Part model, mm, in its own coordinate system. A direction names the side the tool comes from. Coordinates: 2 decimals unless noted, no trailing zeros. Order: outer loops, then holes, each group sorted by start corner. A loop starts at its lowest first (then second) coordinate and runs counter-clockwise, first axis right, second up.
1) Cut at A-A (x = 0). List the corners of the cut face in (y, z).
2) Mould opens along Z. For faces 4 (the flat face through (4, -1, -9)), 5 (the cylindrical face through (-1.73, 2.03, 7.81)), 6 (the cylindrical face through (11.923, 1.535, 3.755)) say: +Z half, -Z half, draft (parallel to the pull), parting line (faces both ways), or undercut.
3) Cut at D-D (z = -3.25). List the corners of the cut face in (x, y), and give its area (3 significant figures).
4) Pin check, flat tips, straight feed: pin 1 Ø1.6 at (x, z) = (-9, -6.5) entering from +Y; pin 2 Ø9.5 at (x, z) = (0, 0) entering from -Y; pin 3 Ø3 at (x, y) = (4.5, 3) entering from -Z; pin 4 Ø2 at (y, z) = (3, 3.5) entering from +X. Stop position of each tip, or through.
5) Tool access for faces 1 (the flat face through (11, 0, 0)), 2 (the flat face through (-0.2, 4, 8.2)), 3 (the flat face through (-2, 0, -8)): list every direction of +Z, -Z, +X, -X, +Y, -Y with a clear straight run to the whole face (end or side of a thin tool).
6) Cut at B-B (z = 0). List the corners of the cut face in (x, y), and give its area (3 significant figures).
7) Wall check: L1, parallel to X at y = 1.95, z = 0; L2, parallel to Z at x = 0, y = 2.25; L3, parallel to X at y = 0.8, z = -0.75. Give the ranges that are in metal, low to high.
8) Cut at C-C (y = 0.35). List the corners of the cut face in (x, z).
```python
from build123d import *

# Parameters (mm, degrees)
SKETCH_1_R          = 12.5
EXTRUDE_1_DEPTH     = 4
SKETCH_2_R          = 1
EXTRUDE_2_DEPTH     = 7.5
SKETCH_5_R          = 6
CUT_EXTRUDE_1_DEPTH = 10
SKETCH_7_R          = 1
CUT_EXTRUDE_2_DEPTH = 7.5
SKETCH_8_R          = 12.5
SKETCH_8_R_2        = 6
CUT_EXTRUDE_3_DEPTH = 10
SKETCH_9_R          = 1
EXTRUDE_3_DEPTH     = 10
SKETCH_10_R         = 1
CUT_EXTRUDE_4_DEPTH = 14
SKETCH_11_R         = 8
CUT_EXTRUDE_5_DEPTH = 10
SKETCH_13_R         = 12.5
SKETCH_13_R_2       = 9.6
EXTRUDE_5_DEPTH     = 1


with BuildPart() as part:
    # 草图1 → 凸台-拉伸1 (new body)
    with BuildSketch(Plane(origin=(0, 0, 0), x_dir=(1, 0, 0), z_dir=(0, 1, 0))):
        Circle(SKETCH_1_R)
    extrude(amount=EXTRUDE_1_DEPTH)

    # 草图2 → 凸台-拉伸2 (add)
    with BuildSketch(Plane(origin=(0, 4, 0), x_dir=(1, 0, 0), z_dir=(0, 1, 0))):
        with Locations((10, 0)):
            Circle(SKETCH_2_R)
        with Locations((3.399186938, -10.461621679)):
            Circle(SKETCH_2_R)
        with Locations((-8.590169944, -7.416694292)):
            Circle(SKETCH_2_R)
        with Locations((-9.399186938, 4.926796007)):
            Circle(SKETCH_2_R)
        with Locations((2.090169944, 9.510565163)):
            Circle(SKETCH_2_R)
    extrude(amount=EXTRUDE_2_DEPTH)

    # 草图5 → 切除-拉伸1 (cut)
    with BuildSketch(Plane(origin=(0, 4, 0), x_dir=(1, 0, 0), z_dir=(0, 1, 0))):
        Circle(SKETCH_5_R)
    extrude(amount=-CUT_EXTRUDE_1_DEPTH, mode=Mode.SUBTRACT)

    # 草图7 → 切除-拉伸2 (cut)
    with BuildSketch(Plane(origin=(0, 11.5, 0), x_dir=(1, 0, 0), z_dir=(0, 1, 0))):
        with Locations((-9.399186938, 4.926796007)):
            Circle(SKETCH_7_R)
    extrude(amount=-CUT_EXTRUDE_2_DEPTH, mode=Mode.SUBTRACT)

    # 草图8 → 切除-拉伸3 (cut)
    with BuildSketch(Plane(origin=(0, 4, 0), x_dir=(1, 0, 0), z_dir=(0, 1, 0))):
        Circle(SKETCH_8_R)
        Circle(SKETCH_8_R_2, mode=Mode.SUBTRACT)
    extrude(amount=CUT_EXTRUDE_3_DEPTH, mode=Mode.SUBTRACT)

    # 草图9 → 凸台-拉伸3 (add)
    with BuildSketch(Plane(origin=(0, 4, 0), x_dir=(1, 0, 0), z_dir=(0, 1, 0))):
        with Locations((11, 0)):
            Circle(SKETCH_9_R)
        with Locations((3.399186938, -10.461621679)):
            Circle(SKETCH_9_R)
        with Locations((-8.899186938, -6.465637775)):
            Circle(SKETCH_9_R)
        with Locations((-8.899186938, 6.465637775)):
            Circle(SKETCH_9_R)
        with Locations((3.399186938, 10.461621679)):
            Circle(SKETCH_9_R)
    extrude(amount=EXTRUDE_3_DEPTH)

    # 草图10 → 切除-拉伸4 (cut)
    with BuildSketch(Plane(origin=(0, 14, 0), x_dir=(1, 0, 0), z_dir=(0, 1, 0))):
        with Locations((-8.899186938, -6.465637775)):
            Circle(SKETCH_10_R)
        with Locations((3.399186938, -10.461621679)):
            Circle(SKETCH_10_R)
        with Locations((11, 0)):
            Circle(SKETCH_10_R)
        with Locations((3.399186938, 10.461621679)):
            Circle(SKETCH_10_R)
        with Locations((-8.899186938, 6.465637775)):
            Circle(SKETCH_10_R)
    extrude(amount=-CUT_EXTRUDE_4_DEPTH, mode=Mode.SUBTRACT)

    # 草图11 → 切除-拉伸5 (cut)
    with BuildSketch(Plane(origin=(0, 4, 0), x_dir=(1, 0, 0), z_dir=(0, 1, 0))):
        Circle(SKETCH_11_R)
    extrude(amount=-CUT_EXTRUDE_5_DEPTH, mode=Mode.SUBTRACT)

    # 草图13 → 凸台-拉伸5 (add)
    with BuildSketch(Plane.XZ):
        Circle(SKETCH_13_R)
        Circle(SKETCH_13_R_2, mode=Mode.SUBTRACT)
    extrude(amount=EXTRUDE_5_DEPTH)


solid = part.part
```
Geometry check:
1. outline: (-1, -12.5) - (4, -12.5) - (4, -8) - (0, -8) - (0, -9.6) - (-1, -9.6) - close; (-1, 9.6) - (0, 9.6) - (0, 8) - (4, 8) - (4, 12.5) - (-1, 12.5) - close
2. face 4: draft
2. face 5: undercut
2. face 6: parting line
3. outline: (-12.07, -1) - (-9.03, -1) - (-9.03, 0) - (-7.31, 0) - (-7.31, 4) - (-12.07, 4) - close; (7.31, 0) - (9.03, 0) - (9.03, -1) - (12.07, -1) - (12.07, 4) - (7.31, 4) - close
3. area: 44.2 mm2
4. pin 1: stops at y = 0
4. pin 2: passes through
4. pin 3: stops at z = -12.13
4. pin 4: stops at x = 12.25
5. face 1: +Y
5. face 2: +Z, -Z, +X, -X, +Y
5. face 3: -Y
6. outline: (-12.5, -1) - (-9.6, -1) - (-9.6, 0) - (-8, 0) - (-8, 4) - (-12.5, 4) - close; (8, 0) - (9.6, 0) - (9.6, -1) - (12.5, -1) - (12.5, 4) - (12, 4) - (12, 0) - (10, 0) - (10, 4) - (8, 4) - close
6. area: 33.8 mm2
7. L1: x = -12.5 to -8, 8 to 10, 12 to 12.5
7. L2: z = -12.5 to -8, 8 to 12.5
7. L3: x = -12.48 to -7.96, 7.96 to 10.34, 11.66 to 12.48
8. outline: circle Ø25 at (0, 0); hole circle Ø2 at (-8.9, -6.47); hole circle Ø2 at (-8.9, 6.47); hole circle Ø16 at (0, 0); hole circle Ø2 at (3.4, -10.46); hole circle Ø2 at (3.4, 10.46); hole circle Ø2 at (11, 0)
